```python
from build123d import *

# Parameters (mm, degrees)
SKETCH1_W           = 1066.8
SKETCH1_H           = 1397
BOSS_EXTRUDE1_DEPTH = 6.35


with BuildPart() as part:
    # Sketch1 → Boss-Extrude1 (new body)
    with BuildSketch(Plane(origin=(6993.279954705, 0, -6693.457613122), x_dir=(0.6914509803921883, 0, 0.722423381207088), z_dir=(-0.722423381207088, 0, 0.6914509803921883))):
        with Locations((-1547.448135129, 704.85)):
            Rectangle(SKETCH1_W, SKETCH1_H)
        with BuildLine():
            Line((-1242.648135129, 685.8), (-1852.248135129, 685.8))
            ThreePointArc((-1852.248135129, 685.8), (-1861.22839125, 682.080256121), (-1864.948135129, 673.1))
            Line((-1864.948135129, 673.1), (-1864.948135129, 476.25))
            ThreePointArc((-1864.948135129, 476.25), (-1861.22839125, 467.269743879), (-1852.248135129, 463.55))
            Line((-1852.248135129, 463.55), (-1242.648135129, 463.55))
            ThreePointArc((-1242.648135129, 463.55), (-1233.667879008, 467.269743879), (-1229.948135129, 476.25))
            Line((-1229.948135129, 476.25), (-1229.948135129, 673.1))
            ThreePointArc((-1229.948135129, 673.1), (-1233.667879008, 682.080256121), (-1242.648135129, 685.8))
        make_face(mode=Mode.SUBTRACT)
    extrude(amount=-BOSS_EXTRUDE1_DEPTH)


solid = part.part
```
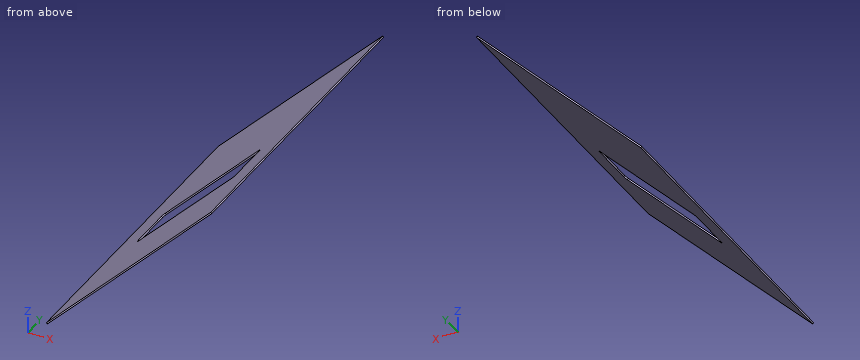
Geometry: final body of the model. Coordinates: model frame, mm. Give positions to 0.01 mm unless a question says otherwise; leave off trailing zeros. Loops run counter-clockwise (first coordinate to the right, second up) from the corner with the lowest first, then second, coordinate; pieces in that order, holes last. Notation, with made-up numbers: (-31, 58) -> (22, 58) arc R18 cw to (22, 65) -> close; hole circle Ø7 at (36.25, 58). An arc over 180 degrees is marked (long way). Return JSON: item names as keys, results as strings.
Item 1: Section B-B, the plane x = 5955. Output: boundary loops of the cut face in (y, z).
Filled in:
{"outline": "(6.35, -7787.43) -> (463.55, -7787.43) -> (463.55, -7778.25) -> (6.35, -7778.25) -> close; (685.8, -7787.43) -> (1403.35, -7787.43) -> (1403.35, -7778.25) -> (685.8, -7778.25) -> close"}
Item 2: Section A-A, the plane z = -7817.5. Output: boundary loops of the cut face in (x, y), plus the area to 3 significant figures.
Filled in:
{"outline": "(5917.43, 6.35) -> (5926.22, 6.35) -> (5926.22, 463.55) -> (5917.43, 463.55) -> close; (5917.43, 685.8) -> (5926.22, 685.8) -> (5926.22, 1403.35) -> (5917.43, 1403.35) -> close", "area": "10,300 mm^2"}
Item 3: Line query: line 1 (X direction, y = 1100, z = -7919.5); line 2 (X direction, y = 188, z = -7998.5); line 3 (Z direction, x = 5695, y = 1189.5). Output: solid intervals per line, ascending.
Filled in:
{"line 1": "5819.8 to 5828.59", "line 2": "5744.19 to 5752.98", "line 3": "-8059.08 to -8049.89"}
Item 4: Section D-D, the plane x = 5629.5. Output: boundary loops of the cut face in (y, z), plus the area to 3 significant figures.
Filled in:
{"outline": "(6.35, -8127.51) -> (1403.35, -8127.51) -> (1403.35, -8118.33) -> (6.35, -8118.33) -> close", "area": "12,800 mm^2"}
Item 5: Pin query (flat end, axial travel): P1, Ø1, axis at y = 839.5, z = -7687.5, coming from the +X side; P2, Ø10, axis at x = 5800.5, y = 286, coming from the +Z side; P3, Ø12, axis at x = 6160.5, y = 779, coming from the -Z side. Return the tip coordinate at first contact, or that it passes through.
Filled in:
{"P1": "x = 6051.12", "P2": "z = -7934.44", "P3": "z = -7578.99"}
Item 6: Section C-C, the plane y = 1056.5. Output: boundary loops of the cut face in (x, z).
Filled in:
{"outline": "(5554.48, -8196.71) -> (5559.06, -8201.1) -> (6296.7, -7430.42) -> (6292.12, -7426.03) -> close"}
